Autodesk Fusion 360 part; units mm, degrees
sketch "Sketch1" plane through (0, 0, 0) normal (0, 1, 0) x (1, 0, 0)
  line L0 (0, 10.6457) -> (2.025, 10.6457)
  line L1 (2.025, 10.6457) -> (2.025, 20.6457)
  line L2 (-2.025, 10.6457) -> (-2.025, 20.6457)
  line L3 (0, 10.6457) -> (-2.025, 10.6457)
  line L4 (-9.4989, 5.2156) -> (-19.0095, 8.3058)
  line L5 (-10.7504, 1.3638) -> (-20.261, 4.454)
  line L6 (-10.1247, 3.2897) -> (-10.7504, 1.3638)
  line L7 (-10.1247, 3.2897) -> (-9.4989, 5.2156)
  line L8 (-7.8957, -7.4223) -> (-13.7735, -15.5125)
  line L9 (-4.6191, -9.8028) -> (-10.497, -17.893)
  line L10 (-6.2574, -8.6126) -> (-4.6191, -9.8028)
  line L11 (-6.2574, -8.6126) -> (-7.8957, -7.4223)
  line L12 (4.6191, -9.8028) -> (10.497, -17.893)
  line L13 (7.8957, -7.4223) -> (13.7735, -15.5125)
  line L14 (6.2574, -8.6126) -> (7.8957, -7.4223)
  line L15 (6.2574, -8.6126) -> (4.6191, -9.8028)
  line L16 (10.7504, 1.3638) -> (20.261, 4.454)
  line L17 (9.4989, 5.2156) -> (19.0095, 8.3058)
  line L18 (10.1247, 3.2897) -> (9.4989, 5.2156)
  line L19 (10.1247, 3.2897) -> (10.7504, 1.3638)
  line L20 (-24.2705, -7.886) -> (-13.7735, -15.5125)
  line L21 (-10.497, -17.893) -> (0, -25.5195)
  line L22 (-15, 20.6457) -> (-19.0095, 8.3058)
  line L23 (-20.261, 4.454) -> (-24.2705, -7.886)
  line L24 (15, 20.6457) -> (2.025, 20.6457)
  line L25 (-2.025, 20.6457) -> (-15, 20.6457)
  line L26 (24.2705, -7.886) -> (20.261, 4.454)
  line L27 (19.0095, 8.3058) -> (15, 20.6457)
  line L28 (0, -25.5195) -> (10.497, -17.893)
  line L29 (13.7735, -15.5125) -> (24.2705, -7.886)
  dimension "d9" = 360
extrude "Extrude1" add sketch "Sketch1" along normal blind 4.3
fillet "Fillet1" radius 4.5 10 edges at (-2.025, 2.15, -20.6457) (2.025, 2.15, -20.6457) (19.0095, 2.15, -8.3058) (20.261, 2.15, -4.454) (10.497, 2.15, 17.893) (13.7735, 2.15, 15.5125) (-19.0095, 2.15, -8.3058) (-20.261, 2.15, -4.454) (-13.7735, 2.15, 15.5125) (-10.497, 2.15, 17.893)
sketch "Sketch2" plane through (0, 4.3, 0) normal (0, 1, 0) x (-1, 0, 0)
  arc A0 (7.852, 14.2524) -> (6.8564, 20.538) centre (4.2114, 16.8975) ccw
  line L0 (6.8564, 20.538) -> (0, 25.5195)
  line L1 (0, 25.5195) -> (-6.8564, 20.538)
  arc A1 (-6.8564, 20.538) -> (-7.852, 14.2524) centre (-4.2114, 16.8975) ccw
  line L2 (-7.852, 14.2524) -> (-4.6191, 9.8028)
  line L3 (-4.6191, 9.8028) -> (-7.8957, 7.4223)
  line L4 (-7.8957, 7.4223) -> (-11.1285, 11.8719)
  arc A2 (-11.1285, 11.8719) -> (-17.4141, 12.8674) centre (-14.7691, 9.2269) ccw
  line L5 (-17.4141, 12.8674) -> (-24.2705, 7.886)
  line L6 (-24.2705, 7.886) -> (-21.6516, -0.1742)
  arc A3 (-21.6516, -0.1742) -> (-15.9813, -3.0634) centre (-17.3718, 1.2163) ccw
  line L7 (-15.9813, -3.0634) -> (-10.7504, -1.3638)
  line L8 (-10.7504, -1.3638) -> (-9.4989, -5.2156)
  line L9 (-9.4989, -5.2156) -> (-14.7297, -6.9152)
  arc A4 (-14.7297, -6.9152) -> (-17.6189, -12.5855) centre (-13.3392, -11.1949) ccw
  line L10 (-17.6189, -12.5855) -> (-15, -20.6457)
  line L11 (-15, -20.6457) -> (-6.525, -20.6457)
  arc A5 (-6.525, -20.6457) -> (-2.025, -16.1457) centre (-6.525, -16.1457) ccw
  line L12 (-2.025, -16.1457) -> (-2.025, -10.6457)
  line L13 (-2.025, -10.6457) -> (2.025, -10.6457)
  line L14 (2.025, -10.6457) -> (2.025, -16.1457)
  arc A6 (2.025, -16.1457) -> (6.525, -20.6457) centre (6.525, -16.1457) ccw
  line L15 (6.525, -20.6457) -> (15, -20.6457)
  line L16 (15, -20.6457) -> (17.6189, -12.5855)
  arc A7 (17.6189, -12.5855) -> (14.7297, -6.9152) centre (13.3392, -11.1949) ccw
  line L17 (14.7297, -6.9152) -> (9.4989, -5.2156)
  line L18 (9.4989, -5.2156) -> (10.7504, -1.3638)
  line L19 (10.7504, -1.3638) -> (15.9813, -3.0634)
  arc A8 (15.9813, -3.0634) -> (21.6516, -0.1742) centre (17.3718, 1.2163) ccw
  line L20 (21.6516, -0.1742) -> (24.2705, 7.886)
  line L21 (24.2705, 7.886) -> (17.4141, 12.8674)
  arc A9 (17.4141, 12.8674) -> (11.1285, 11.8719) centre (14.7691, 9.2269) ccw
  line L22 (11.1285, 11.8719) -> (7.8957, 7.4223)
  line L23 (7.8957, 7.4223) -> (4.6191, 9.8028)
  line L24 (4.6191, 9.8028) -> (7.852, 14.2524)
equation "thickness = 4.3 mm"
equation "notch_depth = 7 mm"
equation "length = 30 mm"
equation "kerf = 0.25 mm"
equation "d10 = thickness"
Can you work these out from the model? Positions are in its coordinate system, mm. A direction names the side the tool comes from. Give positions to 0.01 mm unless a question says otherwise; leave off trailing zeros. Write each loop counter-clockwise with the first axis right and the second up, starting at its lowest first coordinate (ties: lowest second). Pieces come first, ordered by that corner, then holes. Notation, with made-up numbers: M 47,-10.75 L 69,-10.75 A18 ccw 69,-1.75 Z; hole C -13,-11.5 d11. An arc over 180 degrees is marked long. Answer in a Markdown table with one row per item. Add a question column.
Item 1: On a 3-axis mill with a long thin cutter (end or side, diameter ignored), from which of +Z, -Z, +X, -X, +Y, -Y can I reach the whole of each face in a straight line? I mean faces 1 (the cylindrical face through (-3.308, 2.18, -19.293)), 2 (the flat face through (-13.33, 2.12, -2.2)), 3 (the flat face through (-12.078, 2.12, -6.054)). Say none if no direction works.
Item 2: Imagine slicing it at D-D, the plane x = 19. Write out the boundary of the cut face in (y, z), plus the area to 3 significant figures.
Item 3: Imagine slicing it at A-A, the plane x = -12. Write out the boundary of the cut face in (y, z).
Item 4: Please list where these lines run through material, in increasing order: L1, parallel to Z at x = -11, y = 0.8; L2, parallel to Z at x = 11.5, y = 3.5; L3, parallel to X at y = 2.7, z = -16.5.
Item 5: For pin 1 Ø1.5 at (y, z) = (3, 16) entering from -X; pin 2 Ø2 at (y, z) = (2, -14.5) entering from -X; pin 3 Ø2 at (y, z) = (2, -13.5) entering from +X, each with a flat end and sliding along its axis, tell me the tip position at first contact or that it passes through.
Item 6: Imagine slicing it at C-C, the plane x = 13. Write out the boundary of the cut face in (y, z), plus the area to 3 significant figures.
Item 7: We'd pull the mould along X, two halves only. Please class faces 4 (the flat face through (2.025, 2, -13)), 5 (the flat face through (12.078, 2.12, -6.054)), 6 (the cylindrical face through (-17.371, 2.18, -9.196)), 7 (the flat face through (0, 2, -10.646)): released by +X, released by -X, zero draft, split by the parting line, or undercut.
Item 8: Imagine slicing it at B-B, the plane z = 10.5. Write out the boundary of the cut face in (x, y).
Evaluation:
| question | item | result |
|---|---|---|
| 1 | face 1 | -Z, +Y, -Y |
| 1 | face 2 | +Y, -Y |
| 1 | face 3 | -X, +Y, -Y |
| 2 | outline | M 0,-2.98 L 4.3,-2.98 L 4.3,11.72 L 0,11.72 Z |
| 2 | area | 63.2 mm² |
| 3 | outline | M 0,-20.65 L 4.3,-20.65 L 4.3,-6.03 L 0,-6.03 Z; M 0,-1.77 L 4.3,-1.77 L 4.3,12.77 L 0,12.77 Z |
| 4 | L1 | z = -20.65 to -5.7, -1.44 to 11.7 |
| 4 | L2 | z = -20.65 to -5.87, -1.61 to 12.32 |
| 4 | L3 | x = -16.35 to -2.04, 2.04 to 16.35 |
| 5 | pin 1 | stops at x = -8.71 |
| 5 | pin 2 | stops at x = -17.32 |
| 5 | pin 3 | stops at x = 17.65 |
| 6 | outline | M 0,-20.65 L 4.3,-20.65 L 4.3,-6.35 L 0,-6.35 Z; M 0,-2.09 L 4.3,-2.09 L 4.3,13.36 L 0,13.36 Z |
| 6 | area | 128 mm² |
| 7 | face 4 | undercut |
| 7 | face 5 | released by +X |
| 7 | face 6 | released by -X |
| 7 | face 7 | undercut |
| 8 | outline | M -20.67,0 L -10.13,0 L -10.13,4.3 L -20.67,4.3 Z; M -5.13,0 L 5.13,0 L 5.13,4.3 L -5.13,4.3 Z; M 10.13,0 L 20.67,0 L 20.67,4.3 L 10.13,4.3 Z |
